```python
from build123d import *

# Parameters (mm, degrees)
F0_W     = 82.55
F0_H     = 9.525
F1_DEPTH = 3
F2_W     = 77.55
F2_H     = 4.525
F3_DEPTH = 1


with BuildPart() as f1:
    # F0 (on Top) → F1 (new body)
    with BuildSketch(Plane.XY):
        Polygon((-41.275, -4.7625), (-41.275, 4.7625), (-41.275, 7.9375), (-57.15, 7.9375), (-57.15, -7.9375), (-41.275, -7.9375), align=None)
        Rectangle(F0_W, F0_H)
    extrude(amount=F1_DEPTH)

    # F2 (on face) → F3 (cut)
    with BuildSketch(Plane.XY.offset(3)):
        Rectangle(F2_W, F2_H)
    extrude(amount=-F3_DEPTH, mode=Mode.SUBTRACT)


solid = f1.part
```
Source: CAD feature listing. Evaluate the final solid. Frame: model axes, mm. A direction names the side the tool comes from. Round coordinates to 2 decimals unless told otherwise and drop trailing zeros. Write each loop counter-clockwise with the first axis right and the second up, starting at its lowest first coordinate (ties: lowest second). Pieces come first, ordered by that corner, then holes. Notation, with made-up numbers: M -17,9 L 16,9 A14 cw 16,28 Z; hole C 44.5,55.5 d4. An arc over 180 degrees is marked long. Use CSV: the item, a comma, the result in double quotes. Start each with the question number.
Q1. Access query for faces 4 (the face through (-49, 7.938, 1)), 5 (the face through (-41.275, 6, 1)), 6 (the face through (-1, -4.762, 1)). Directions: +Z, -Z, +X, -X, +Y, -Y. A direction counts if a zero-diameter tool reaches every point of the face in a straight line with its end or side. Return the directions, or none.
Q2. Cut plane A-A on y = -0.5. Output: boundary loops of the cut face in (x, z) (3 decimals), plus the area to 3 significant figures.
Q3. Line query: line 1 (X direction, y = 1.75, z = 2.95) (3 decimals); line 2 (Y direction, x = -13.5, z = 2.2); line 3 (Y direction, x = 23.5, z = 1). Output: solid intervals per line, ascending. Write a range as from..to.
Q4. First-contact query: P1, Ø1.5, axis at x = 12.5, z = 2.5, coming from the -Y side; P2, Ø5, axis at x = 3, y = -0.5, coming from the +Z side; P3, Ø1.5, axis at y = -6, z = 1.5, coming from the +X side (3 decimals); P4, Ø0.9, axis at x = 13.5, z = 1.5, coming from the +Y side. Flat tips, straight axial feed; report the tip coordinate or a pass-through.
Q5. Cut plane B-B on x = -27.5. Output: boundary loops of the cut face in (y, z).
Q6. Pull-direction query (Y, two-part tool) for faces 1 (the face through (-1, 4.762, 1)), 2 (the face through (-1, 0, 2)), 3 (the face through (-49, -7.938, 1)); classes: +Y half, -Y half, draft (parallel to the pull), parting line (faces both ways), or undercut.
Results found:
1,face 4,"+Z, -Z, +X, -X, +Y"
1,face 5,"+Z, -Z, +X, +Y"
1,face 6,"+Z, -Z, +X, -Y"
2,outline,"M -57.15,0 L 41.275,0 L 41.275,3 L 38.775,3 L 38.775,2 L -38.775,2 L -38.775,3 L -57.15,3 Z"
2,area,"218 mm^2"
3,line 1,"-57.15..-38.775, 38.775..41.275"
3,line 2,"-4.76..-2.26, 2.26..4.76"
3,line 3,"-4.76..4.76"
4,P1,"y = -4.76"
4,P2,"z = 3"
4,P3,"x = -41.275"
4,P4,"y = 4.76"
5,outline,"M -4.76,0 L 4.76,0 L 4.76,3 L 2.26,3 L 2.26,2 L -2.26,2 L -2.26,3 L -4.76,3 Z"
6,face 1,"+Y half"
6,face 2,"undercut"
6,face 3,"-Y half"
